```python
from build123d import *

# Parameters (mm, degrees)
SKETCH1_R               = 3.3235
BASENUT_DEPTH           = 6.8
ENDCHAMFER_SIZE         = 0.6765
ENDCHAMFER_SIZE2        = 0.390577457
ENDCHAMFER_PART_2_SIZE  = 0.6765
ENDCHAMFER_PART_2_SIZE2 = 0.390577457


with BuildPart() as part:
    # Sketch1 → BaseNut (new body)
    with BuildSketch(Plane.XY):
        Polygon((7.505553499, 0), (3.75277675, 6.5), (-3.75277675, 6.5), (-7.505553499, 0), (-3.75277675, -6.5), (3.75277675, -6.5), align=None)
        Circle(SKETCH1_R, mode=Mode.SUBTRACT)
    extrude(amount=-BASENUT_DEPTH)

    # Sketch2 → Double-Chamfer (revolve, cut)
    with BuildSketch(Plane(origin=(0, 0, 0), x_dir=(1, 0, 0), z_dir=(0, 1, 0))):
        Polygon((-7.505553499, 6.8), (-6.125, 6.8), (-7.505553499, 6.002937065), align=None)
        Polygon((-7.505553499, 0.797062935), (-7.505553499, 0), (-6.125, 0), align=None)
    revolve(axis=Axis((0, 0, -3.375940562), (0, 0, 1)), mode=Mode.SUBTRACT)

    # EndChamfer
    endchamfer_edges = [part.edges().sort_by_distance(p)[0] for p in [
        (-3.3235, 0, -6.8),
    ]]
    endchamfer_side = [part.faces().sort_by_distance(p)[0] for p in [
        (-3.3235, 0, -3.4),
    ]]
    chamfer(endchamfer_edges, length=ENDCHAMFER_SIZE, length2=ENDCHAMFER_SIZE2, reference=endchamfer_side[0])

    # EndChamfer part 2
    endchamfer_part_2_edges = [part.edges().sort_by_distance(p)[0] for p in [
        (-3.3235, 0, 0),
    ]]
    endchamfer_part_2_side = [part.faces().sort_by_distance(p)[0] for p in [
        (5.951758839, 0, 0),
    ]]
    chamfer(endchamfer_part_2_edges, length=ENDCHAMFER_PART_2_SIZE, length2=ENDCHAMFER_PART_2_SIZE2, reference=endchamfer_part_2_side[0])


solid = part.part
```
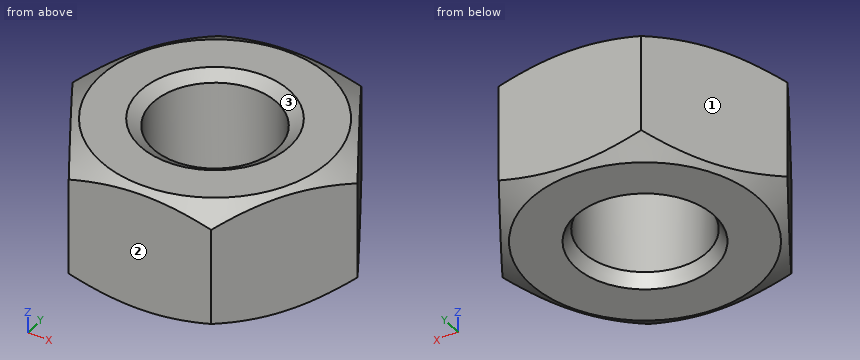
For this review, take the finished solid that the model builds, in its own axes (mm). Face numbers are marked on the shaded views. Give positions to 0.01 mm unless a question says otherwise; leave off trailing zeros. Write each loop counter-clockwise with the first axis right and the second up, starting at its lowest first coordinate (ties: lowest second). Pieces come first, ordered by that corner, then holes. Notation, with made-up numbers: M 25,88.5 L 39,88.5 A24 ccw 39,124.5 Z; hole C 75,-2 d8. An arc over 180 degrees is marked long. One line per item, written item: value.
1) Take a section at B-B, the plane z = -4.5. Write out the cut boundary in (x, y).
Results are:
outline: M -7.51,0 L -3.75,-6.5 L 3.75,-6.5 L 7.51,0 L 3.75,6.5 L -3.75,6.5 Z; hole C 0,0 d6.65
2) The part is to be moulded in two halves that separate along X. For the marked faces 1, 2 and 3, say which applies: +X half, -X half, draft (parallel to the pull), parting line (faces both ways), or undercut.
Results are:
face 1: -X half
face 2: draft
face 3: undercut
3) Take a section at A-A, the plane x = 0. Write out the cut boundary in (y, z) (1 decimal), then the cut area to 3 significant figures.
Results are:
outline: M -6.5,-6.6 L -6.1,-6.8 L -3.7,-6.8 L -3.3,-6.1 L -3.3,-0.4 L -4,0 L -6.1,0 L -6.5,-0.2 Z; M 3.3,-6.1 L 3.7,-6.8 L 6.1,-6.8 L 6.5,-6.6 L 6.5,-0.2 L 6.1,0 L 4,0 L 3.3,-0.4 Z
area: 42.5 mm²
4) For P1, Ø4, axis at x = 3, y = 2.5, coming from the +Z side; P2, Ø1.5, axis at y = 4, z = -2.5, coming from the +X side, all flat-tipped, find the tip position at first contact; note any pin that passes through.
Results are:
P1: stops at z = 0
P2: stops at x = 5.63
5) For line 1 (Y direction, x = 0, z = -2.35); line 2 (X direction, y = -1, z = -4); line 3 (X direction, y = -0.25, z = -5.25), list the stretches that pass through material, from the lowest coordinate up. Write a range as from..to.
Results are:
line 1: y = -6.5..-3.32, 3.32..6.5
line 2: x = -6.93..-3.17, 3.17..6.93
line 3: x = -7.36..-3.31, 3.31..7.36
